Here's how the part is built. I have some questions about the finished solid (model axes, mm). A direction names the side the tool comes from. Coordinates: 2 decimals unless noted, no trailing zeros. Write each loop counter-clockwise with the first axis right and the second up, starting at its lowest first coordinate (ties: lowest second). Pieces come first, ordered by that corner, then holes.
Item 1: For faces 4 (the face through (-755.65, -370, -131)), 5 (the face through (-850.9, -57, -160)), 6 (the face through (835, -57, -279.4)), 7 (the face through (819.15, -57, -229)), which set-ups out of +Z, -Z, +X, -X, +Y, -Y let a thin tool reach every point of the face, with its end or its side?
Item 2: I'm going to push flat-ended pins straight in: P1, Ø21, axis at y = -729, z = -172.5, coming from the -X side; P2, Ø1.5, axis at x = 422.5, z = 120, coming from the +Y side; P3, Ø9.5, axis at x = -779.5, y = -725, coming from the -Z side; P4, Ø8, axis at x = -252, z = -111, coming from the -Y side. Where does each tip first touch, or does it pass through?
Item 3: If we mould it in two halves opening along X, with no side actions, what happens to faces 1 (the face through (-835, -57, -38.1)), 2 (the face through (-819.15, -396, -131)), 3 (the face through (755.65, -370, -131))? For each: pulls with the +X half, pulls with the -X half, needs draft (parallel to the pull), parting line crosses it, or undercut.
Item 4: I want a section at C-C (z = 213). Please give me the cut outline in (x, y), and give its area (3 significant figures).
Item 5: I want a section at D-D (x = 696). Please give me the cut outline in (y, z), and give its area (3 significant figures).
Item 6: I want a section at B-B (y = -294). Please give me the cut outline in (x, z).
Item 7: I want a section at A-A (z = -198). Please give me the cut outline in (x, y), and give its area (3 significant figures).
Item 8: Please list where these lines run through material, in increasing order: line 1 (X direction, y = -611.5, z = -83); line 2 (Y direction, x = -781.5, z = 80); line 3 (Y direction, x = 400, z = -237).
from build123d import *

# Parameters (mm, degrees)
SKETCH1_W           = 1828.8
SKETCH1_H           = 762
BOSS_EXTRUDE1_DEPTH = 31.75
SKETCH2_W           = 31.75
SKETCH2_H           = 241.3
BOSS_EXTRUDE2_DEPTH = 50.8
SKETCH3_W           = 63.5
SKETCH3_H           = 95.25
BOSS_EXTRUDE3_DEPTH = 685.8
SKETCH4_W           = 76.2
SKETCH4_H           = 711.2
BOSS_EXTRUDE4_DEPTH = 19.05


with BuildPart() as part:
    # Sketch1 → Boss-Extrude1 (new body)
    with BuildSketch(Plane(origin=(0, 0, 0), x_dir=(1, 0, 0), z_dir=(0, 1, 0))):
        Rectangle(SKETCH1_W, SKETCH1_H)
    extrude(amount=-BOSS_EXTRUDE1_DEPTH)

    # Sketch2 → Boss-Extrude2 (add)
    with BuildSketch(Plane.XZ.offset(31.75)):
        with Locations((-835.025, -158.75)):
            Rectangle(SKETCH2_W, SKETCH2_H)
    boss_extrude2 = extrude(amount=BOSS_EXTRUDE2_DEPTH)

    # Sketch3 → Boss-Extrude3 (add)
    with BuildSketch(Plane.XZ.offset(31.75)):
        with Locations((-787.4, -130.175)):
            Rectangle(SKETCH3_W, SKETCH3_H)
    boss_extrude3 = extrude(amount=BOSS_EXTRUDE3_DEPTH)

    # Sketch4 → Boss-Extrude4 (add)
    with BuildSketch(Plane.XZ.offset(717.55)):
        with Locations((-787.4, 0)):
            Rectangle(SKETCH4_W, SKETCH4_H)
    boss_extrude4 = extrude(amount=BOSS_EXTRUDE4_DEPTH)

    # Mirror1: Boss-Extrude2, Boss-Extrude3, Boss-Extrude4 across plane
    add(boss_extrude2.mirror(Plane(origin=(0, 0, 0), x_dir=(0, 0, 1), z_dir=(1, 0, 0))))
    add(boss_extrude3.mirror(Plane(origin=(0, 0, 0), x_dir=(0, 0, 1), z_dir=(1, 0, 0))))
    add(boss_extrude4.mirror(Plane(origin=(0, 0, 0), x_dir=(0, 0, 1), z_dir=(1, 0, 0))))


solid = part.part
Answer:
1. face 4: +Z, -Z
1. face 5: +Z, -Z, -X, -Y
1. face 6: -Z, +X, -X
1. face 7: -Z
2. P1: stops at x = -825.5
2. P2: stops at y = 0
2. P3: stops at z = -355.6
2. P4: stops at y = -31.75
3. face 1: needs draft
3. face 2: pulls with the -X half
3. face 3: undercut
4. outline: (-914.4, -31.75) - (914.4, -31.75) - (914.4, 0) - (-914.4, 0) - close; (-825.5, -736.6) - (-749.3, -736.6) - (-749.3, -717.55) - (-825.5, -717.55) - close; (749.3, -736.6) - (825.5, -736.6) - (825.5, -717.55) - (749.3, -717.55) - close
4. area: 61,000 mm2
5. outline: (-31.75, -381) - (0, -381) - (0, 381) - (-31.75, 381) - close
5. area: 24,200 mm2
6. outline: (-819.15, -177.8) - (-755.65, -177.8) - (-755.65, -82.55) - (-819.15, -82.55) - close; (755.65, -177.8) - (819.15, -177.8) - (819.15, -82.55) - (755.65, -82.55) - close
7. outline: (-914.4, -31.75) - (-850.9, -31.75) - (-850.9, -82.55) - (-819.15, -82.55) - (-819.15, -31.75) - (819.15, -31.75) - (819.15, -82.55) - (850.9, -82.55) - (850.9, -31.75) - (914.4, -31.75) - (914.4, 0) - (-914.4, 0) - close; (-825.5, -736.6) - (-749.3, -736.6) - (-749.3, -717.55) - (-825.5, -717.55) - close; (749.3, -736.6) - (825.5, -736.6) - (825.5, -717.55) - (749.3, -717.55) - close
7. area: 64,200 mm2
8. line 1: x = -819.15 to -755.65, 755.65 to 819.15
8. line 2: y = -736.6 to -717.55, -31.75 to 0
8. line 3: y = -31.75 to 0
